Verification items for the finished model (mm, model axes). A direction names the side the tool comes from. Give positions to 0.01 mm unless a question says otherwise; leave off trailing zeros. Write each loop counter-clockwise with the first axis right and the second up, starting at its lowest first coordinate (ties: lowest second). Pieces come first, ordered by that corner, then holes.
from build123d import *

# Parameters (mm, degrees)
F0_W     = 37.211
F0_H     = 39.37
F1_DEPTH = 4.191
F2_W     = 35.56
F2_H     = 6.858
F3_DEPTH = 39.37
F4_R     = 0.76199


# Not quite as in the source:
# - a fillet or chamfer is up to 0.001 mm smaller than in the source, because OpenCascade refuses the exact size


with BuildPart() as f1:
    # F0 (on Front) → F1 (new body, symmetric)
    with BuildSketch(Plane.XZ):
        Rectangle(F0_W, F0_H)
    extrude(amount=F1_DEPTH, both=True)

    # F2 (on face) → F3 (cut)
    with BuildSketch(Plane.XY.offset(19.685)):
        Rectangle(F2_W, F2_H)
    extrude(amount=-F3_DEPTH, mode=Mode.SUBTRACT)

    # F4 (radius 0.762 in the source; OpenCascade refuses exactly that, so slightly less here)
    f4_edges = [f1.edges().sort_by_distance(p)[0] for p in [
        (0, -4.191, -19.685),
        (18.6055, 0, -19.685),
        (0, 4.191, -19.685),
        (-18.6055, 0, -19.685),
    ]]
    fillet(f4_edges, radius=F4_R)


solid = f1.part
Item 1: Set-up check for faces 5 (the face through (18.606, 0, 0)), 6 (the face through (0, 3.429, 0)): record each of +Z, -Z, +X, -X, +Y, -Y from which the full face is reachable in a straight line by a thin tool's end or side.
Answer key:
face 5: +Z, -Z, +X, +Y, -Y
face 6: +Z, -Z
Item 2: Scan lines: line 1 along Y through (x, z) = (0, -18); line 2 along X through (y, z) = (-0.5, -4); line 3 along Z through (x, y) = (-10, -3.5) (3 decimals). Record each from-to range of solid material in increasing order.
Answer key:
line 1: y = -4.19 to -3.43, 3.43 to 4.19
line 2: x = -18.61 to -17.78, 17.78 to 18.61
line 3: z = -19.682 to 19.685
Item 3: Release check for a two-part mould opening along Y. For faces 1 (the face through (0, -3.429, 0)), 2 (the face through (-17.78, 0, 0)), 3 (the face through (-18.606, 0, 0)), 4 (the face through (0, -4.191, 1)) record: released by +Y, released by -Y, zero draft, split by the parting line, or undercut.
Answer key:
face 1: undercut
face 2: undercut
face 3: zero draft
face 4: released by -Y
Item 4: Sectioned sample at C-C on z = -13. Record the cut outline in (x, y).
Answer key:
outline: (-18.61, -4.19) - (18.61, -4.19) - (18.61, 4.19) - (-18.61, 4.19) - close; hole (-17.78, -3.43) - (17.78, -3.43) - (17.78, 3.43) - (-17.78, 3.43) - close
